Check sheet for the modelled part. Datum: model origin and axes. Units: mm. A direction names the side the tool comes from. Round coordinates to 2 decimals unless told otherwise and drop trailing zeros. Loops run counter-clockwise (first coordinate to the right, second up) from the corner with the lowest first, then second, coordinate; pieces in that order, holes last. Notation, with made-up numbers: (69.25, 4.25) - (116.25, 4.25) arc R21 cw to (116.25, 9.25) - close; hole circle Ø10 at (46, 42). An arc over 180 degrees is marked (long way). Return JSON: item names as keys, results as strings.
from build123d import *

# Parameters (mm, degrees)
SKETCH3_R           = 0.25
CUT_EXTRUDE1_DEPTH  = 4
SKETCH4_R           = 0.75
SKETCH4_R_2         = 0.25
BOSS_EXTRUDE1_DEPTH = 1


with BuildPart() as part:
    # Sketch1 → Revolve1 (revolve)
    with BuildSketch(Plane.XY):
        Polygon((0.927471423, 4.5), (1.927471423, 4.5), (1.927471423, 1), (-2.072528577, 1), (-2.072528577, 3), (0.927471423, 3.5), align=None)
    revolve(axis=Axis((-11.471189379, 0, 0), (1, 0, 0)))

    # Sketch3 → Cut-Extrude1 (cut)
    with BuildSketch(Plane.ZY.offset(2.072528577)):
        with Locations((0, 1.974515761)):
            Circle(SKETCH3_R)
    extrude(amount=-CUT_EXTRUDE1_DEPTH, mode=Mode.SUBTRACT)

    # Sketch4 → Boss-Extrude1 (add)
    with BuildSketch(Plane.ZY.offset(2.072528577)):
        with Locations((0, 1.974515761)):
            Circle(SKETCH4_R)
        with Locations((0, 1.974515761)):
            Circle(SKETCH4_R_2, mode=Mode.SUBTRACT)
    extrude(amount=BOSS_EXTRUDE1_DEPTH)


solid = part.part
Q1. Scan lines: probe 1 along X at (y, z) = (-2.5, 1); probe 2 along Z at (x, y) = (1.15, 0); probe 3 along X at (y, z) = (-2.75, 2.75). Record each from-to range of solid material in increasing order. Write a range as [from, to].
Answer key:
{"probe 1": "x = [-2.07, 1.93]", "probe 2": "z = [-4.5, -1], [1, 4.5]", "probe 3": "x = [0.93, 1.93]"}
Q2. Sectioned sample at B-B (z = 0). Enter the section's corners in (x, y).
Answer key:
{"outline": "(-3.07, 1.22) - (-2.07, 1.22) - (-2.07, 1) - (1.93, 1) - (1.93, 1.72) - (-3.07, 1.72) - close; (-3.07, 2.22) - (1.93, 2.22) - (1.93, 4.5) - (0.93, 4.5) - (0.93, 3.5) - (-2.07, 3) - (-2.07, 2.72) - (-3.07, 2.72) - close; (-2.07, -3) - (0.93, -3.5) - (0.93, -4.5) - (1.93, -4.5) - (1.93, -1) - (-2.07, -1) - close"}
Q3. Draft check along Y on faces 1 (the face through (1.43, -0.59, 4.46)), 2 (the face through (-2.073, -1.3, 0)), 3 (the face through (0, 0, -1)). Enter one of: released by +Y, released by -Y, zero draft, split by the parting line, or undercut.
Answer key:
{"face 1": "split by the parting line", "face 2": "zero draft", "face 3": "undercut"}
Q4. Sectioned sample at C-C (x = 0.8). Enter the section's corners in (y, z), plus the area to 3 significant figures.
Answer key:
{"outline": "circle Ø6.96 at (0, 0); hole circle Ø2 at (0, 0); hole circle Ø0.5 at (1.97, 0)", "area": "34.7 mm²"}
Q5. Sectioned sample at D-D (x = -0.15). Enter the section's corners in (y, z), plus the area to 3 significant figures.
Answer key:
{"outline": "circle Ø6.64 at (0, 0); hole circle Ø2 at (0, 0); hole circle Ø0.5 at (1.97, 0)", "area": "31.3 mm²"}
Q6. Sectioned sample at A-A (y = 0). Enter the section's corners in (x, z), plus the area to 3 significant figures.
Answer key:
{"outline": "(-2.07, -3) - (0.93, -3.5) - (0.93, -4.5) - (1.93, -4.5) - (1.93, -1) - (-2.07, -1) - close; (-2.07, 1) - (1.93, 1) - (1.93, 4.5) - (0.93, 4.5) - (0.93, 3.5) - (-2.07, 3) - close", "area": "20.5 mm²"}
Q7. Tool access check on faces 4 (the face through (1.927, 1, -1)), 5 (the face through (-2.57, 1.24, -0.16)). Record the directions out of +Z, -Z, +X, -X, +Y, -Y that give a thin tool (end or side, any length) a straight path to the whole face; none if there is none.
Answer key:
{"face 4": "+Z, -Z, +X, +Y, -Y", "face 5": "-X"}
Q8. Depth check by flat-ended pin: P1, Ø3, axis at y = -1, z = 0.5, coming from the -X side. Enter the tip coordinate at first touch or a pass-through.
Answer key:
{"P1": "stops at x = -2.07"}
